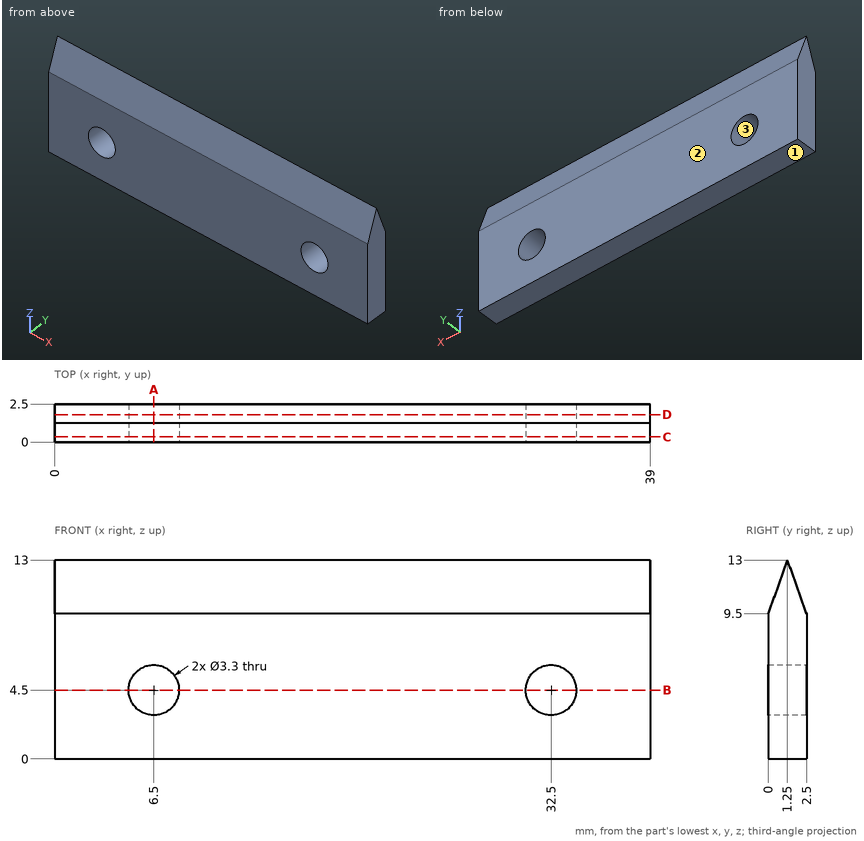
Design review of the part shown in the three views and the two pictorial views. Dimensions are in mm from the part's minimum x, y and z. Round coordinates to 2 decimals unless told otherwise and drop trailing zeros. Loops run counter-clockwise (first coordinate to the right, second up) from the corner with the lowest first, then second, coordinate; pieces in that order, holes last. Notation, with made-up numbers: M -37,58 L 18,58 A27 ccw 18,87 Z; hole C 36,87 d4. An arc over 180 degrees is marked long. Write item = value, one per line.
Item 1: Take a section at D-D on y = 1.8. Write out the cut boundary in (x, z).
Return value:
outline = M 0,0 L 39,0 L 39,11.46 L 0,11.46 Z; hole C 6.5,4.5 d3.3; hole C 32.5,4.5 d3.3
Item 2: Take a section at C-C on y = 0.35. Write out the cut boundary in (x, z).
Return value:
outline = M 0,0 L 39,0 L 39,10.48 L 0,10.48 Z; hole C 6.5,4.5 d3.3; hole C 32.5,4.5 d3.3
Item 3: Insertion check: P1, Ø4.5, axis at x = 6.5, z = 4.5, coming from the -Y side; P2, Ø3, axis at x = 13.5, z = 11.5, coming from the +Y side. Each pin has a flat end and moves straight along its axis. Give the tip position at first contact, or say it passes through.
Return value:
P1 = 0
P2 = 2.32
Item 4: Take a section at B-B on z = 4.5. Write out the cut boundary in (x, y), then the cut area to 3 significant figures.
Return value:
outline = M 0,0 L 4.85,0 L 4.85,2.5 L 0,2.5 Z; M 8.15,0 L 30.85,0 L 30.85,2.5 L 8.15,2.5 Z; M 34.15,0 L 39,0 L 39,2.5 L 34.15,2.5 Z
area = 81.0 mm2
Item 5: For line 1 (X direction, y = 0.85, z = 4.5); line 2 (X direction, y = 0.8, z = 5.75); line 3 (Y direction, x = 19, z = 10), list the stretches that pass through material, from the lowest coordinate up. Write a range as [from, to].
Return value:
line_1 = [0, 4.85], [8.15, 30.85], [34.15, 39]
line_2 = [0, 5.42], [7.58, 31.42], [33.58, 39]
line_3 = [0.18, 2.32]
Item 6: The part is to be moulded in two halves that separate along Z. For the marked faces 1, 2 and 3, say which applies: released by +Z, released by -Z, zero draft, split by the parting line, or undercut.
Return value:
face_1 = released by -Z
face_2 = zero draft
face_3 = undercut
Item 7: Take a section at A-A on x = 6.5. Write out the cut boundary in (y, z), then the cut area to 3 significant figures.
Return value:
outline = M 0,0 L 2.5,0 L 2.5,2.85 L 0,2.85 Z; M 0,6.15 L 2.5,6.15 L 2.5,9.5 L 1.25,13 L 0,9.5 Z
area = 19.9 mm2
